The listing builds one solid part. Answer for the finished solid, in the listing's coordinates (mm). Face numbers are marked on the shaded views. A direction names the side the tool comes from. Coordinates: 2 decimals unless noted, no trailing zeros. Order: outer loops, then holes, each group sorted by start corner. A loop starts at its lowest first (then second) coordinate and runs counter-clockwise, first axis right, second up. Notation, with made-up numbers: (69.5, 6) -> (108.5, 6) arc R35 cw to (108.5, 39) -> close; hole circle Ø4 at (43, 57). An arc over 180 degrees is marked (long way). Return JSON: item names as keys, results as strings.
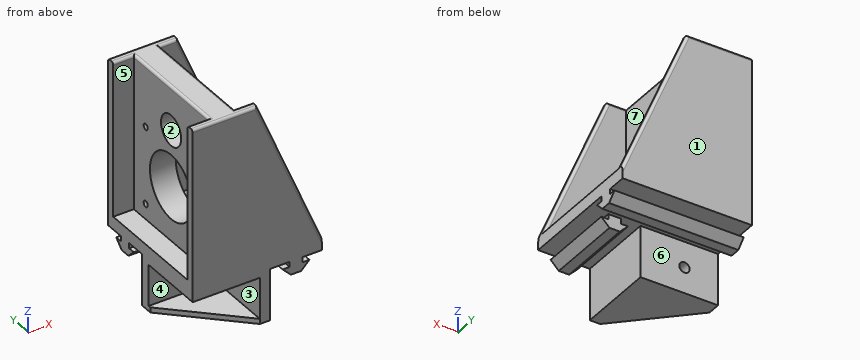
from build123d import *

# Parameters (mm, degrees)
SKETCH_W        = 50
SKETCH_H        = 85
PAD_DEPTH       = 50
POCKET_DEPTH    = 50
POCKET001_DEPTH = 30
SKETCH004_W     = 16
SKETCH004_H     = 26
POCKET002_DEPTH = 26
SKETCH005_R     = 2
POCKET003_DEPTH = 4
POCKET005_DEPTH = 4
SKETCH008_W     = 44
SKETCH008_H     = 60
POCKET006_DEPTH = 32
SKETCH009_R     = 12.5
SKETCH009_R_2   = 5.95
SKETCH009_R_3   = 1.19841
POCKET007_DEPTH = 18.001
SKETCH010_W     = 44
SKETCH010_H     = 60
POCKET008_DEPTH = 8
POCKET009_DEPTH = 50.001
FILLET_R        = 1


with BuildPart() as part:
    # Sketch → Pad (new body)
    with BuildSketch(Plane.YZ):
        Rectangle(SKETCH_W, SKETCH_H)
    extrude(amount=PAD_DEPTH)

    # Sketch001 (on Face6 of Pad) → Pocket (cut)
    with BuildSketch(Plane.YZ.offset(50)):
        Polygon((5, -22.5), (5, -42.5), (25, -42.5), (25, -22.5), (17.48396, -22.5), (17.48396, -24.5), (20.18396, -24.5), (17, -27.68), (13, -27.68), (9.81604, -24.5), (12.51604, -24.5), (12.51604, -22.5), align=None)
    extrude(amount=-POCKET_DEPTH, mode=Mode.SUBTRACT)

    # Sketch003 (on Face2 of Pocket) → Pocket001 (cut)
    with BuildSketch(Plane(origin=(0, -25, 0), x_dir=(0, 0, -1), z_dir=(0, -1, 0))):
        Polygon((42.5, 50), (22.5, 50), (22.5, 42.48), (24.5, 42.48), (24.5, 45.18), (27.68, 42), (27.68, 38), (24.5, 34.82), (24.5, 37.52), (22.5, 37.52), (22.5, 30), (42.5, 30), align=None)
    extrude(amount=-POCKET001_DEPTH, mode=Mode.SUBTRACT)

    # Sketch004 (on Face2 of Pocket001) → Pocket002 (cut)
    with BuildSketch(Plane(origin=(0, -25, 0), x_dir=(0, 0, -1), z_dir=(0, -1, 0))):
        with Locations((32.5, 13)):
            Rectangle(SKETCH004_W, SKETCH004_H)
    extrude(amount=-POCKET002_DEPTH, mode=Mode.SUBTRACT)

    # Sketch005 (on Face30 of Pocket002) → Pocket003 (cut)
    with BuildSketch(Plane(origin=(0, 1, 0), x_dir=(0, 0, -1), z_dir=(0, -1, 0))):
        with Locations((32.5, 13)):
            Circle(SKETCH005_R)
    extrude(amount=-POCKET003_DEPTH, mode=Mode.SUBTRACT)

    # Sketch007 → Pocket005 (cut)
    with BuildSketch(Plane.YX.offset(42.5)):
        Polygon((-25.002718, 26), (-25, 0), (0, 0), align=None)
    extrude(amount=-POCKET005_DEPTH, mode=Mode.SUBTRACT)

    # Sketch008 (on Face5 of Pocket005) → Pocket006 (cut)
    with BuildSketch(Plane.YZ.offset(50)):
        with Locations((0, 12.5)):
            Rectangle(SKETCH008_W, SKETCH008_H)
    extrude(amount=-POCKET006_DEPTH, mode=Mode.SUBTRACT)

    # Sketch009 (on Face6 of Pocket006) → Pocket007 (cut, through all)
    with BuildSketch(Plane.YZ.offset(18)):
        with Locations((0, 3.5)):
            Circle(SKETCH009_R)
        with Locations((0, 25.5)):
            Circle(SKETCH009_R_2)
        with Locations((-15, 18.5)):
            Circle(SKETCH009_R_3)
        with Locations((-15, -11.5)):
            Circle(SKETCH009_R_3)
        with Locations((15, -11.5)):
            Circle(SKETCH009_R_3)
        with Locations((15, 18.5)):
            Circle(SKETCH009_R_3)
    extrude(amount=-POCKET007_DEPTH, mode=Mode.SUBTRACT)

    # Sketch010 (on Face2 of Pocket007) → Pocket008 (cut)
    with BuildSketch(Plane(origin=(0, 0, 0), x_dir=(0, 1, 0), z_dir=(-1, 0, 0))):
        with Locations((0, -12.5)):
            Rectangle(SKETCH010_W, SKETCH010_H)
    extrude(amount=-POCKET008_DEPTH, mode=Mode.SUBTRACT)

    # Sketch011 (on Face11 of Pocket008) → Pocket009 (cut, through all)
    with BuildSketch(Plane(origin=(0, -25, 0), x_dir=(0, 0, -1), z_dir=(0, -1, 0))):
        Polygon((-42.5, 50), (-42.5, 25), (17.5, 50), align=None)
    extrude(amount=-POCKET009_DEPTH, mode=Mode.SUBTRACT)

    # Fillet
    fillet_edges = [part.edges().sort_by_distance(p)[0] for p in [
        (8, 0, 42.5),
        (12.5, -25, 42.5),
        (4, -22, 42.5),
        (12.5, 25, 42.5),
        (37.5, 22, 12.5),
        (37.5, 25, 12.5),
        (18, 0, 42.5),
        (21.5, 22, 42.5),
        (21.5, -22, 42.5),
        (4, 22, 42.5),
        (37.5, -25, 12.5),
        (37.5, -22, 12.5),
    ]]
    fillet(fillet_edges, radius=FILLET_R)


solid = part.part
1. The part is cut by section B-B on x = 13. Give the number of separate pieces and of enclosed holes in the cut face, and give its area (3 significant figures).
Answer block:
{"separate pieces": "2", "enclosed holes": "6", "area": "2,810 mm2"}
2. The part is cut by section D-D on y = -7. Give the vertices of the cut face in (x, z).
Answer block:
{"outline": "(0, -24.5) -> (26, -24.5) -> (26, -40.5) -> (7.28, -40.5) -> (7.28, -42.5) -> (30, -42.5) -> (30, -22.5) -> (37.52, -22.5) -> (37.52, -24.5) -> (34.82, -24.5) -> (38, -27.68) -> (42, -27.68) -> (45.18, -24.5) -> (42.48, -24.5) -> (42.48, -22.5) -> (50, -22.5) -> (50, -17.5) -> (18, -17.5) -> (18, -6.86) -> (8, -6.86) -> (8, -17.5) -> (0, -17.5) -> close; (8, 13.86) -> (18, 13.86) -> (18, 41.5) arc R1 ccw to (17, 42.5) -> (9, 42.5) arc R1 ccw to (8, 41.5) -> close"}
3. The part is cut by section A-A on z = -32.5. Give the vertices of the cut face in (x, y).
Answer block:
{"outline": "(0, 1) -> (11, 1) -> (11, 5) -> (0, 5) -> close; (15, 1) -> (26, 1) -> (26, -25) -> (30, -25) -> (30, 5) -> (15, 5) -> close"}
4. Determine the mould class of the marked faces 1, 2, 3 and 4 for opening direction Y: pulls with the +Y half, pulls with the -Y half, needs draft (parallel to the pull), parting line crosses it, or undercut.
Answer block:
{"face 1": "pulls with the +Y half", "face 2": "undercut", "face 3": "needs draft", "face 4": "pulls with the -Y half"}
5. Each of these flat-tipped pins is pushed along its axis until it touches: pin 1 Ø1.2 at (x, y) = (41, -14.5) entering from -Z; pin 2 Ø1 at (y, z) = (-13, 16) entering from -X; pin 3 Ø4 at (x, y) = (33.5, 4) entering from +Z. Where does it stop, or does it pass through?
Answer block:
{"pin 1": "stops at z = -27.68", "pin 2": "stops at x = 8", "pin 3": "stops at z = -17.5"}
6. For the marked faces 5, 6 and 7, determine the directions among +Z, -Z, +X, -X, +Y, -Y from which every point of the face is accessible in a straight line to the end or side of a thin tool.
Answer block:
{"face 5": "+Z, -X", "face 6": "-Z, +X, -X", "face 7": "+Z, +X"}
7. Consider line 1 (Z direction, x = 13, y = 0); line 2 (Z direction, x = 12.25, y = 15); line 3 (Y direction, x = 32.5, z = 19.5). Determine where each line is inside the solid, lowest interval first. Write a range as from..to.
Answer block:
{"line 1": "z = -42.5..-40.5, -24.5..-9, 16..19.55, 31.45..42.5", "line 2": "z = -27.68..-12.7, -10.3..17.3, 19.7..42.5", "line 3": "y = -25..-22, 22..25"}
